Autodesk Inventor part; units mm, degrees
ref_plane "Work Plane1" through (0, 0, 53.975) normal (0, 0, 1) x (1, 0, 0)
ref_plane "Work Plane2" through (53.975, 0, 0) normal (1, 0, 0) x (0, 1, 0)
ref_plane "XZ Plane" through (0, 0, 0) normal (0, 1, 0) x (-1, 0, 0)
sketch "Sketch1" plane through (0, 0, 0) normal (0, 1, 0) x (-1, 0, 0)
  circle A0 centre (0, 0) radius 47.625
  circle A1 centre (0, 0) radius 53.975
  dimension "d0" = 95.25
  dimension "d1" = 107.95
extrude "Extrusion1" add sketch "Sketch1" along normal mid plane 25.4
ref_plane "Work Plane1" through (0, 0, 53.975) normal (0, 0, 1) x (1, 0, 0)
sketch "Sketch2" plane through (0, 0, 53.975) normal (0, 0, 1) x (1, 0, 0)
  point P0 (0, 0)
  point P1 (0, 0)
hole "Hole1" at (0, 0, 53.975) direction (0, 0, -1) diameter 6.35 end through all
ref_plane "Work Plane2" through (53.975, 0, 0) normal (1, 0, 0) x (0, 1, 0)
sketch "Sketch3" plane through (53.975, 0, 0) normal (1, 0, 0) x (0, 1, 0)
  point P0 (0, 0)
  point P1 (0, 0)
hole "Hole2" at (53.975, 0, 0) direction (-1, 0, 0) diameter 6.7564 end through all
equation "\"d0\" = innerDiam"
equation "\"d1\" = outerRingDism"
equation "\"d2\" = ringHeight"
equation "\"d5\" = ringAxelDiam"
equation "\"innerDiam\" = 95.25"
equation "\"ringThickness\" = 6.35"
equation "\"ringHeight\" = 25.4"
equation "\"ringAxelDiam\" = 6.35"
equation "\"outerRingDism\" = innerDiam + 2 * ringThickness"
equation "\"outerRingRadius\" = 0.5 * outerRingDism"
equation "\"d4\" = outerRingRadius"
equation "\"d12\" = outerRingRadius"
properties part number "outerRing"
Geometry check sheet. Reference: the model listing, model coordinates, mm. Round coordinates to 2 decimals unless told otherwise and drop trailing zeros. Order: outer loops, then holes, each group sorted by start corner. A loop starts at its lowest first (then second) coordinate and runs counter-clockwise, first axis right, second up. Notation, with made-up numbers: M 19,-27 L 74,-27 A13 cw 74,-13 Z; hole C -19,-19.5 d2. An arc over 180 degrees is marked long. Answer in a Markdown table with one row per item.
(1) Go/stop test with flat-tipped pins: P1, Ø4, axis at y = -8.5, z = 15, coming from the -X side; P2, Ø5, axis at y = 6.5, z = -30, coming from the -X side; P3, Ø2, axis at y = -10, z = -20.5, coming from the -X side. Record where each tip stops, or that it passes through.
Responses:
| item | result |
|---|---|
| P1 | stops at x = -52.39 |
| P2 | stops at x = -46.44 |
| P3 | stops at x = -50.33 |
(2) Scan lines: probe 1 along Y at (x, z) = (0, -50) (3 decimals); probe 2 along Z at (x, y) = (0, -3.5) (3 decimals); probe 3 along Z at (x, y) = (-3, 5.75). Record each from-to range of solid material in increasing order. Write a range as from..to.
Responses:
| item | result |
|---|---|
| probe 1 | y = -12.7..-3.175, 3.175..12.7 |
| probe 2 | z = -53.975..-47.625, 47.625..53.975 |
| probe 3 | z = -53.89..-47.53, 47.53..53.89 |
(3) Sectioned sample at B-B, the plane x = 0. Record the cut outline in (y, z) (3 decimals).
Responses:
| item | result |
|---|---|
| outline | M -12.7,-53.975 L -3.175,-53.975 L -3.175,-47.625 L -12.7,-47.625 Z; M -12.7,47.625 L -3.175,47.625 L -3.175,53.975 L -12.7,53.975 Z; M 3.175,-53.975 L 12.7,-53.975 L 12.7,-47.625 L 3.175,-47.625 Z; M 3.175,47.625 L 12.7,47.625 L 12.7,53.975 L 3.175,53.975 Z |
(4) Sectioned sample at A-A, the plane z = 0. Record the cut outline in (x, y) (3 decimals).
Responses:
| item | result |
|---|---|
| outline | M -53.975,-12.7 L -47.625,-12.7 L -47.625,-3.378 L -53.975,-3.378 Z; M -53.975,3.378 L -47.625,3.378 L -47.625,12.7 L -53.975,12.7 Z; M 47.625,-12.7 L 53.975,-12.7 L 53.975,-3.378 L 47.625,-3.378 Z; M 47.625,3.378 L 53.975,3.378 L 53.975,12.7 L 47.625,12.7 Z |
(5) Draft check along Y on faces 1 (the face through (3.1, 0.69, -50.79)), 2 (the face through (0, 12.7, -48)), 3 (the face through (0, -12.7, -48)). Enter one of: released by +Y, released by -Y, zero draft, split by the parting line, or undercut.
Responses:
| item | result |
|---|---|
| face 1 | undercut |
| face 2 | released by +Y |
| face 3 | released by -Y |
(6) Sectioned sample at D-D, the plane x = 42. Record the cut outline in (y, z).
Responses:
| item | result |
|---|---|
| outline | M -12.7,-33.9 L 12.7,-33.9 L 12.7,-22.45 L -12.7,-22.45 Z; M -12.7,22.45 L 12.7,22.45 L 12.7,33.9 L -12.7,33.9 Z |
(7) Sectioned sample at C-C, the plane z = 37.5. Record the cut outline in (x, y), and give its area (3 significant figures).
Responses:
| item | result |
|---|---|
| outline | M -38.82,-12.7 L -29.36,-12.7 L -29.36,12.7 L -38.82,12.7 Z; M 29.36,-12.7 L 38.82,-12.7 L 38.82,12.7 L 29.36,12.7 Z |
| area | 481 mm² |
